from build123d import *

# Parameters (mm, degrees)
SKETCH1_R           = 20.2311
SKETCH1_R_2         = 13.0175
SKETCH1_W           = 6.35
SKETCH1_H           = 101.1682
SKETCH1_W_2         = 170.072742275
SKETCH1_H_2         = 6.35
BOSS_EXTRUDE1_DEPTH = 6.35


with BuildPart() as part:
    # Sketch1 → Boss-Extrude1 (new body)
    with BuildSketch(Plane.XY):
        with BuildLine():
            Line((-127.583895856, -254.619594065), (67.888846419, -254.619594065))
            ThreePointArc((67.888846419, -254.619594065), (72.378974479, -252.759722126), (74.238846419, -248.269594065))
            Line((74.238846419, -248.269594065), (74.238846419, -121.701394065))
            ThreePointArc((74.238846419, -121.701394065), (72.378974479, -117.211266005), (67.888846419, -115.351394065))
            Line((67.888846419, -115.351394065), (-127.583895856, -115.351394065))
            ThreePointArc((-127.583895856, -115.351394065), (-132.074023916, -117.211266005), (-133.933895856, -121.701394065))
            Line((-133.933895856, -121.701394065), (-133.933895856, -248.269594065))
            ThreePointArc((-133.933895856, -248.269594065), (-132.074023916, -252.759722126), (-127.583895856, -254.619594065))
        make_face()
        with Locations((-49.389995856, -151.457494065)):
            Circle(SKETCH1_R, mode=Mode.SUBTRACT)
        with Locations((19.736104144, -171.688594065)):
            Circle(SKETCH1_R_2, mode=Mode.SUBTRACT)
        with Locations((-75.971095856, -184.985494065)):
            Rectangle(SKETCH1_W, SKETCH1_H, mode=Mode.SUBTRACT)
        with Locations((-124.408895856, -184.985494065)):
            Rectangle(SKETCH1_W, SKETCH1_H, mode=Mode.SUBTRACT)
        with Locations((64.713846419, -184.985494065)):
            Rectangle(SKETCH1_W, SKETCH1_H, mode=Mode.SUBTRACT)
        with Locations((-22.808895856, -184.985494065)):
            Rectangle(SKETCH1_W, SKETCH1_H, mode=Mode.SUBTRACT)
        with Locations((-29.847524719, -124.876394065)):
            Rectangle(SKETCH1_W_2, SKETCH1_H_2, mode=Mode.SUBTRACT)
        with Locations((-29.847524719, -245.094594065)):
            Rectangle(SKETCH1_W_2, SKETCH1_H_2, mode=Mode.SUBTRACT)
    extrude(amount=BOSS_EXTRUDE1_DEPTH)


solid = part.part
Source: CAD feature listing. Evaluate the final solid. Frame: model axes, mm. A direction names the side the tool comes from. Round coordinates to 2 decimals unless told otherwise and drop trailing zeros. Write each loop counter-clockwise with the first axis right and the second up, starting at its lowest first coordinate (ties: lowest second). Pieces come first, ordered by that corner, then holes. Notation, with made-up numbers: M 59.25,-21.75 L 95.25,-21.75 A17 ccw 95.25,9.25 Z; hole C -2.75,-11 d5. An arc over 180 degrees is marked long. One line per item, written item: value. Start each with the question number.
Item 1: Mould query, pull axis Y, two halves, no side actions, for faces 1 (the cylindrical face through (72.428, -117.261, 3.131)), 2 (the flat face through (-133.934, -184, 3)), 3 (the flat face through (-124, -235.57, 3)). Classes: pulls with the +Y half, pulls with the -Y half, needs draft (parallel to the pull), parting line crosses it, or undercut.
Item 2: Ray query, L1, parallel to Y at x = -8.5, z = 3.5; L2, parallel to X at y = -196, z = 3.75; L3, parallel to X at y = -243.5, z = 4.25. Return the intervals inside material, ascending. Write a range as from..to.
Item 3: Pin query (flat end, axial travel): pin 1 (15.5 mm diameter, centred on x = 19.74, y = -171.69, fed in from -Z). Return the tip coordinate at first contact, or that it passes through.
Item 4: Section query A-A (x = 37). Return the cut outline in (y, z), plus the area to 3 significant figures.
Item 5: Section query C-C (y = -168). Return the cut outline in (x, z), plus the area to 3 significant figures.
Item 6: Set-up query: faces 4 (the flat face through (61.539, -186, 3)), 5 (the flat face through (-31, -254.62, 3)). Return all of +Z, -Z, +X, -X, +Y, -Y with unobstructed straight access to the full face (end or side cutting, diameter ignored); none if empty.
Item 7: Section query D-D (z = 3.25). State how many separate pieces and enclosed holes the cut face has, plus the area to 3 significant figures.
Item 8: Section query B-B (y = -217.5). Return the cut outline in (x, z).
Result set:
1. face 1: pulls with the +Y half
1. face 2: needs draft
1. face 3: undercut
2. L1: y = -254.62..-248.27, -241.92..-128.05, -121.7..-115.35
2. L2: x = -133.93..-127.58, -121.23..-79.15, -72.8..-25.98, -19.63..61.54, 67.89..74.24
2. L3: x = -133.93..-114.88, 55.19..74.24
3. pin 1: passes through
4. outline: M -254.62,0 L -248.27,0 L -248.27,6.35 L -254.62,6.35 Z; M -241.92,0 L -128.05,0 L -128.05,6.35 L -241.92,6.35 Z; M -121.7,0 L -115.35,0 L -115.35,6.35 L -121.7,6.35 Z
4. area: 804 mm²
5. outline: M -133.93,0 L -127.58,0 L -127.58,6.35 L -133.93,6.35 Z; M -121.23,0 L -79.15,0 L -79.15,6.35 L -121.23,6.35 Z; M -72.8,0 L -61.04,0 L -61.04,6.35 L -72.8,6.35 Z; M -37.74,0 L -25.98,0 L -25.98,6.35 L -37.74,6.35 Z; M -19.63,0 L 7.25,0 L 7.25,6.35 L -19.63,6.35 Z; M 32.22,0 L 61.54,0 L 61.54,6.35 L 32.22,6.35 Z; M 67.89,0 L 74.24,0 L 74.24,6.35 L 67.89,6.35 Z
5. area: 854 mm²
6. face 4: +Z, -Z
6. face 5: +Z, -Z, +X, -X, -Y
7. separate pieces: 1
7. enclosed holes: 8
7. area: 22,400 mm²
8. outline: M -133.93,0 L -127.58,0 L -127.58,6.35 L -133.93,6.35 Z; M -121.23,0 L -79.15,0 L -79.15,6.35 L -121.23,6.35 Z; M -72.8,0 L -25.98,0 L -25.98,6.35 L -72.8,6.35 Z; M -19.63,0 L 61.54,0 L 61.54,6.35 L -19.63,6.35 Z; M 67.89,0 L 74.24,0 L 74.24,6.35 L 67.89,6.35 Z
